The figure shows three views and two pictorial views of one solid part (mm, origin at its lowest corner). Answer the questions. A direction names the side the tool comes from. Coordinates: 2 decimals unless noted, no trailing zeros. Loops run counter-clockwise (first coordinate to the right, second up) from the corner with the lowest first, then second, coordinate; pieces in that order, holes last. Notation, with made-up numbers: (77, -26.75) - (122, -26.75) arc R21 ccw to (122, -12.75) - close; hole circle Ø3 at (46.5, 43). An arc over 180 degrees is marked (long way). One line per question, with ' | ' between items.
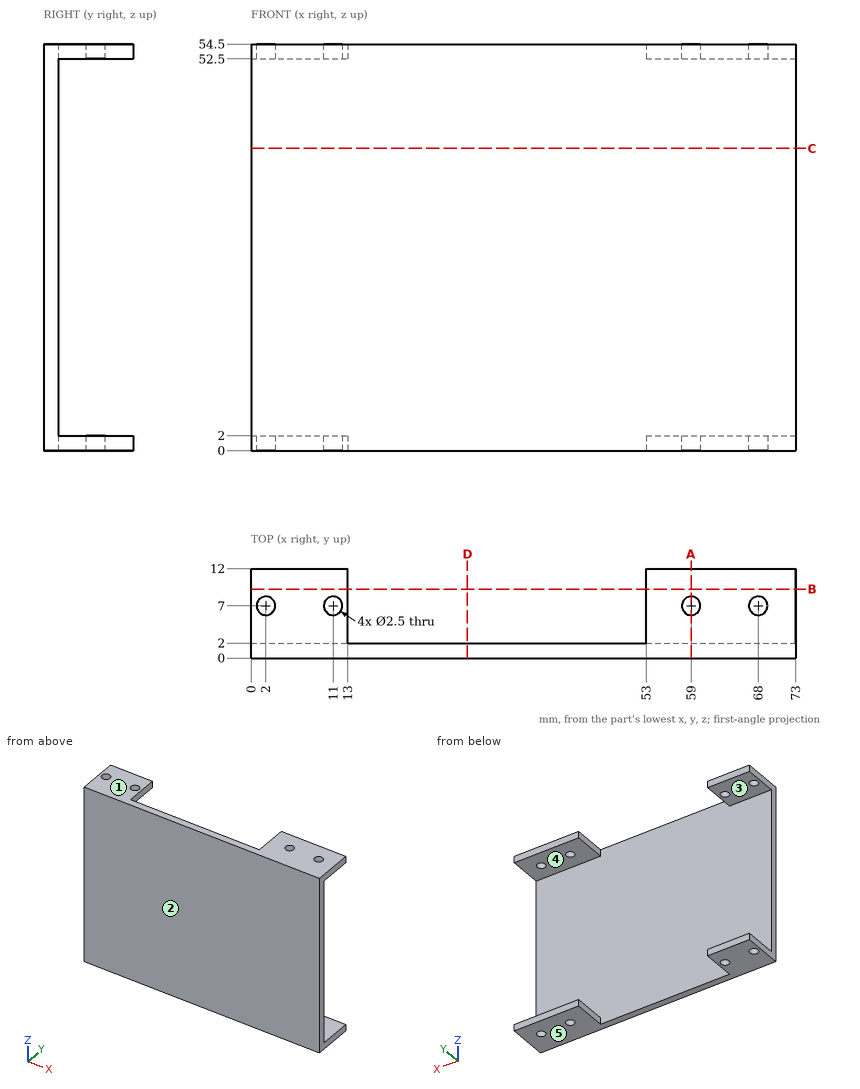
Item 1: Find section D-D, the plane x = 29. Write down the section's boundary in (y, z), plus the area to 3 significant figures.
Taken from the geometry:
outline: (0, 0) - (2, 0) - (2, 54.5) - (0, 54.5) - close | area: 109 mm2
Item 2: Find the intervals of material crossed by line 1 (Z direction, x = 69.5, y = 10); line 2 (Y direction, x = 68, z = 53); line 3 (Y direction, x = 61, z = 23), in increasing order. Write a range as [from, to].
Taken from the geometry:
line 1: z = [0, 2], [52.5, 54.5] | line 2: y = [0, 5.75], [8.25, 12] | line 3: y = [0, 2]
Item 3: Find section B-B, the plane y = 9.25. Write down the section's boundary in (x, z).
Taken from the geometry:
outline: (0, 0) - (13, 0) - (13, 2) - (0, 2) - close; (0, 52.5) - (13, 52.5) - (13, 54.5) - (0, 54.5) - close; (53, 0) - (73, 0) - (73, 2) - (53, 2) - close; (53, 52.5) - (73, 52.5) - (73, 54.5) - (53, 54.5) - close
Item 4: Find section A-A, the plane x = 59. Write down the section's boundary in (y, z), plus the area to 3 significant figures.
Taken from the geometry:
outline: (0, 0) - (5.75, 0) - (5.75, 2) - (2, 2) - (2, 52.5) - (5.75, 52.5) - (5.75, 54.5) - (0, 54.5) - close; (8.25, 0) - (12, 0) - (12, 2) - (8.25, 2) - close; (8.25, 52.5) - (12, 52.5) - (12, 54.5) - (8.25, 54.5) - close | area: 139 mm2
Item 5: Which of the six approach directions +Z, -Z, +X, -X, +Y, -Y give full straight-line access (tool end or side, diameter ignored) to the marked faces 4 and 5?
Taken from the geometry:
face 4: +X, -X, +Y | face 5: -Z, +X, -X, +Y, -Y
Item 6: The mould has two halves that part along Z. Classify the marked faces 1, 2 and 3: pulls with the +Z half, pulls with the -Z half, needs draft (parallel to the pull), parting line crosses it, or undercut.
Taken from the geometry:
face 1: pulls with the +Z half | face 2: needs draft | face 3: undercut
Item 7: Each of these flat-tipped pins is pushed along its axis until it touches: pin 1 Ø3 at (x, y) = (59, 7) entering from -Z; pin 2 Ø2 at (x, y) = (2, 7) entering from -Z; pin 3 Ø16.5 at (x, z) = (54, 38) entering from +Y. Where does it stop, or does it pass through?
Taken from the geometry:
pin 1: stops at z = 0 | pin 2: passes through | pin 3: stops at y = 2
Item 8: Find section C-C, the plane z = 40.5. Write down the section's boundary in (x, y), plus the area to 3 significant figures.
Taken from the geometry:
outline: (0, 0) - (73, 0) - (73, 2) - (0, 2) - close | area: 146 mm2
